Input: part model. Units: mm. Frame: model coordinates. A direction names the side the tool comes from. Give positions to 0.01 mm unless a question says otherwise; leave off trailing zeros. Order: outer loops, then holes, each group sorted by start corner. A loop starts at its lowest first (then second) coordinate and runs counter-clockwise, first axis right, second up. Notation, with made-up numbers: (12, -11.5) - (40, -11.5) arc R24 ccw to (40, 2.5) - close; hole circle Ø1 at (-33, 71.25). An arc over 180 degrees is marked (long way). Use a Markdown table: item, result.
Autodesk Inventor part; units mm, degrees
ref_plane "YZ Plane" through (0, 0, 0) normal (1, 0, 0) x (0, 1, 0)
ref_plane "XZ Plane" through (0, 0, 0) normal (0, 1, 0) x (-1, 0, 0)
ref_plane "XY Plane" through (0, 0, 0) normal (0, 0, 1) x (1, 0, 0)
sketch "Sketch_1" plane through (0, 0, 0) normal (1, 0, 0) x (0, 1, 0)
  arc A0 (-15.55, 7.25) -> (-15.55, -7.25) centre (10.2312, 0) ccw
  line L0 (-15.55, -7.25) -> (15.55, -7.25)
  arc A1 (15.55, -7.25) -> (15.55, 7.25) centre (-10.2312, 0) ccw
  line L1 (15.55, 7.25) -> (-15.55, 7.25)
extrude "Extrusion1" add sketch "Sketch_1" along normal blind 73
sketch "Sketch_8" plane through (0, 0, 0) normal (0, 0, 1) x (1, 0, 0)
  line L0 (0, 0) -> (-3.8, 0)
  line L1 (-3.8, 0) -> (-3.8, 3)
  line L2 (-3.8, 3) -> (-3.271, 6)
  line L3 (-3.271, 6) -> (-2.15, 6)
  line L4 (-2.15, 6) -> (-2.15, 4.36)
  line L5 (-2.15, 4.36) -> (-0.65, 4.36)
  line L6 (-0.65, 4.36) -> (-0.65, 3.4)
  line L7 (-0.65, 3.4) -> (0, 3.4)
  line L8 (0, 3.4) -> (0, 0)
  line L9 (0, 0) -> (-3.8, 0)
revolve "Revolution1" add sketch "Sketch_8" angle 360 about axis through (0, 0, 0) along (1, 0, 0)
sketch "Sketch_2" plane through (0, 0, 0) normal (0, 0, 1) x (1, 0, 0)
  line L0 (4.2, 0) -> (-3.95, 0)
  line L1 (-3.95, 0) -> (-3.95, 3.15)
  line L2 (-3.95, 3.15) -> (-3.8, 3.15)
  arc A0 (-3.8, 3.15) -> (-3.65, 3) centre (-3.65, 3.15) ccw
  line L3 (-3.65, 3) -> (4.2, 3)
  line L4 (4.2, 3) -> (4.2, 0)
  line L5 (4.2, 0) -> (-3.95, 0)
revolve "Revolution2" cut sketch "Sketch_2" angle 360 about axis through (4.2, 0, 0) along (1, 0, 0)
sketch "Sketch_9" plane through (-3.8, 0, 0) normal (1, 0, 0) x (0, 0, -1)
  circle A0 centre (0, 0) radius 7
  arc A1 (-4.9, -0.975) -> (4.9, -0.975) centre (0, -0.975) ccw
  line L0 (4.9, -0.975) -> (4.9, 0.975)
  arc A2 (4.9, 0.975) -> (-4.9, 0.975) centre (0, 0.975) ccw
  line L1 (-4.9, 0.975) -> (-4.9, -0.975)
extrude "Extrusion2" cut sketch "Sketch_9" along normal blind 1.65
sketch "Sketch_10" plane through (-2.15, 0, 0) normal (1, 0, 0) x (0, 1, 0)
  circle A0 centre (0, 0) radius 6
  arc A1 (1.4185, -4.1228) -> (-1.4185, -4.1228) centre (0, 0) ccw
  arc A2 (-1.4185, -4.1228) -> (-1.2558, -4.15) centre (-1.2558, -3.65) ccw
  line L0 (-1.2558, -4.15) -> (1.2558, -4.15)
  arc A3 (1.2558, -4.15) -> (1.4185, -4.1228) centre (1.2558, -3.65) ccw
extrude "Extrusion3" cut sketch "Sketch_10" along normal blind 1.5
sketch "Sketch_3" plane through (0, 0, 0) normal (0, 0, 1) x (1, 0, 0)
  line L0 (76.8, 0) -> (73, 0)
  line L1 (73, 0) -> (73, 3.4)
  line L2 (73, 3.4) -> (73.65, 3.4)
  line L3 (73.65, 3.4) -> (73.65, 4.36)
  line L4 (73.65, 4.36) -> (75.15, 4.36)
  line L5 (75.15, 4.36) -> (75.15, 6)
  line L6 (75.15, 6) -> (76.271, 6)
  line L7 (76.271, 6) -> (76.8, 3)
  line L8 (76.8, 3) -> (76.8, 0)
  line L9 (76.8, 0) -> (73, 0)
revolve "Revolution3" add sketch "Sketch_3" angle 360 about axis through (76.8, 0, 0) along (1, 0, 0)
sketch "Sketch_4" plane through (0, 0, 0) normal (0, 0, 1) x (1, 0, 0)
  line L0 (76.95, 0) -> (68.8, 0)
  line L1 (68.8, 0) -> (68.8, 3)
  line L2 (68.8, 3) -> (76.65, 3)
  arc A0 (76.65, 3) -> (76.8, 3.15) centre (76.65, 3.15) ccw
  line L3 (76.8, 3.15) -> (76.95, 3.15)
  line L4 (76.95, 3.15) -> (76.95, 0)
  line L5 (76.95, 0) -> (68.8, 0)
revolve "Revolution4" cut sketch "Sketch_4" angle 360 about axis through (76.95, 0, 0) along (1, 0, 0)
sketch "Sketch_5" plane through (76.8, 0, 0) normal (1, 0, 0) x (0, 0, -1)
  circle A0 centre (0, 0) radius 7
  arc A1 (-4.9, -0.975) -> (4.9, -0.975) centre (0, -0.975) ccw
  line L0 (4.9, -0.975) -> (4.9, 0.975)
  arc A2 (4.9, 0.975) -> (-4.9, 0.975) centre (0, 0.975) ccw
  line L1 (-4.9, 0.975) -> (-4.9, -0.975)
extrude "Extrusion4" cut sketch "Sketch_5" against normal blind 1.65
sketch "Sketch_11" plane through (75.15, 0, 0) normal (-1, 0, 0) x (0, 1, 0)
  circle A0 centre (0, 0) radius 6
  arc A1 (1.4185, -4.1228) -> (-1.4185, -4.1228) centre (0, 0) ccw
  arc A2 (-1.4185, -4.1228) -> (-1.2558, -4.15) centre (-1.2558, -3.65) ccw
  line L0 (-1.2558, -4.15) -> (1.2558, -4.15)
  arc A3 (1.2558, -4.15) -> (1.4185, -4.1228) centre (1.2558, -3.65) ccw
extrude "Extrusion5" cut sketch "Sketch_11" along normal blind 1.5
sketch "Sketch_6" plane through (30, 0, 0) normal (1, 0, 0) x (0, 0, -1)
  line L0 (-10, -20) -> (10, -20)
  line L1 (10, -20) -> (10, 20)
  line L2 (10, 20) -> (-10, 20)
  line L3 (-10, 20) -> (-10, -20)
  arc A0 (-7.15, -15.45) -> (7.15, -15.45) centre (0, 9.6112) ccw
  line L4 (7.15, -15.45) -> (7.15, 15.45)
  arc A1 (7.15, 15.45) -> (-7.15, 15.45) centre (0, -9.6112) ccw
  line L5 (-7.15, 15.45) -> (-7.15, -15.45)
extrude "Extrusion6" cut sketch "Sketch_6" along normal blind 0.1
sketch "Sketch_7" plane through (63, 0, 0) normal (1, 0, 0) x (0, 0, -1)
  line L0 (-10, -20) -> (10, -20)
  line L1 (10, -20) -> (10, 20)
  line L2 (10, 20) -> (-10, 20)
  line L3 (-10, 20) -> (-10, -20)
  arc A0 (-7.15, -15.45) -> (7.15, -15.45) centre (0, 9.6112) ccw
  line L4 (7.15, -15.45) -> (7.15, 15.45)
  arc A1 (7.15, 15.45) -> (-7.15, 15.45) centre (0, -9.6112) ccw
  line L5 (-7.15, 15.45) -> (-7.15, -15.45)
extrude "Extrusion7" cut sketch "Sketch_7" along normal blind 0.1
properties part number "532624 VN-05-M-I3-PQ2-VQ2-A"
1. Pin query (flat end, axial travel): pin 1 (1.4 mm diameter, centred on x = -2.5, y = 0, fed in from -Z); pin 2 (8 mm diameter, centred on x = 19.5, z = -6, fed in from +Y); pin 3 (5 mm diameter, centred on x = 56, z = -1.5, fed in from -Y). Return the tip coordinate at first contact, or that it passes through.
Response:
| item | result |
|---|---|
| pin 1 | stops at z = -4.9 |
| pin 2 | stops at y = 16.48 |
| pin 3 | stops at y = -16.55 |
2. Material intervals for line 1 along Z through (x, y) = (-1, 0); line 2 along Z through (x, y) = (75.25, 0); line 3 along X through (y, z) = (11.5, -0.25), sorted ascending.
Response:
| item | result |
|---|---|
| line 1 | z = -4.15 to -3, 3 to 4.36 |
| line 2 | z = -4.9 to -3, 3 to 4.9 |
| line 3 | x = 0 to 73 |
3. Section query B-B (x = 35.5). Return loops of the section in (y, z), then the cut area to 3 significant figures.
Response:
| item | result |
|---|---|
| outline | (-15.55, -7.25) - (15.55, -7.25) arc R26.78 ccw to (15.55, 7.25) - (-15.55, 7.25) arc R26.78 ccw to start |
| area | 470 mm^2 |
4. Section query A-A (y = 8.5). Return loops of the section in (x, z), then the cut area to 3 significant figures.
Response:
| item | result |
|---|---|
| outline | (0, -7.25) - (30, -7.25) - (30, -7.15) - (30.1, -7.15) - (30.1, -7.25) - (63, -7.25) - (63, -7.15) - (63.1, -7.15) - (63.1, -7.25) - (73, -7.25) - (73, 7.25) - (63.1, 7.25) - (63.1, 7.15) - (63, 7.15) - (63, 7.25) - (30.1, 7.25) - (30.1, 7.15) - (30, 7.15) - (30, 7.25) - (0, 7.25) - close |
| area | 1,060 mm^2 |
5. Set-up query: faces 4 (the face through (-0.65, -3, 2)), 5 (the face through (-2.808, 5.874, 0.108)), 6 (the face through (73, -3, 0)). Return all of +Z, -Z, +X, -X, +Y, -Y with unobstructed straight access to the full face (end or side cutting, diameter ignored); none if empty.
Response:
| item | result |
|---|---|
| face 4 | none |
| face 5 | -X, +Y |
| face 6 | +X |
6. Mould query, pull axis X, two halves, no side actions, for faces 1 (the face through (-3.754, 3.011, -1.248)), 2 (the face through (67.98, -16.55, -0.1)), 3 (the face through (-2.15, -0.46, -4.33)). Classes: pulls with the +X half, pulls with the -X half, needs draft (parallel to the pull), parting line crosses it, or undercut.
Response:
| item | result |
|---|---|
| face 1 | pulls with the -X half |
| face 2 | needs draft |
| face 3 | undercut |
